from build123d import *

# Parameters (mm, degrees)
LEFT_EXT_DEPTH = 63.5
HOLE_R         = 4.699
HOLE_CUT_DEPTH = 286.961588331


with BuildPart() as part:
    # Left → left_ext (new body)
    with BuildSketch(Plane.XY):
        Polygon((-165.1, 19.05), (-10.998522627, 285.961588331), (10.998522629, 285.961588331), (-143.102954744, 19.05), align=None)
    extrude(amount=LEFT_EXT_DEPTH)

    # hole → hole_cut (cut, through all)
    with BuildSketch(Plane(origin=(0, 0, 0), x_dir=(1, 0, 0), z_dir=(0, 1, 0))):
        with Locations((0, -31.75)):
            Circle(HOLE_R)
    extrude(amount=HOLE_CUT_DEPTH, mode=Mode.SUBTRACT)


solid = part.part
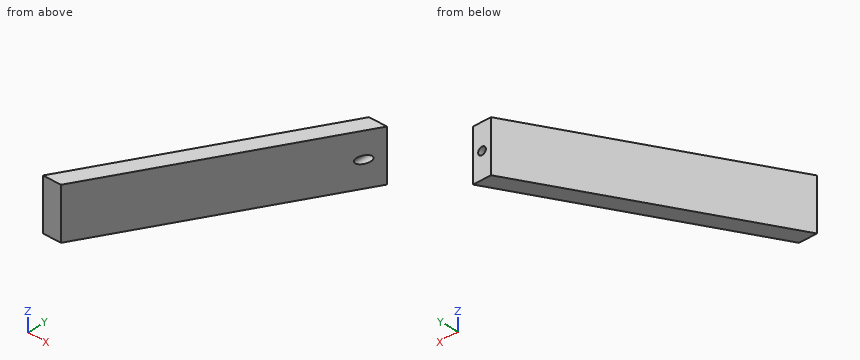
For this review, take the finished solid that the model builds, in its own axes (mm). Coordinates: 2 decimals unless noted, no trailing zeros. Loops run counter-clockwise (first coordinate to the right, second up) from the corner with the lowest first, then second, coordinate; pieces in that order, holes last. Notation, with made-up numbers: (-5, -24.5) - (4, -24.5) arc R38 ccw to (4, 14.5) - close; hole circle Ø5 at (-9, 78.5). An arc over 180 degrees is marked (long way). Return JSON: item names as keys, results as strings.
Item 1: Insertion check: pin 1 (8.5 mm diameter, centred on x = 0, z = 31.75, fed in from -Y); pin 2 (2 mm diameter, centred on y = 233, z = 34, fed in from -X); pin 3 (8 mm diameter, centred on x = -129, z = 27.5, fed in from +Y); pin 4 (4 mm diameter, centred on y = 74.5, z = 13.5, fed in from -X). Each pin has a flat end and moves straight along its axis. Give the tip position at first contact, or say it passes through.
Determined:
{"pin 1": "passes through", "pin 2": "stops at x = -42.15", "pin 3": "stops at y = 88.51", "pin 4": "stops at x = -134.24"}
Item 2: For line 1 (Z direction, x = 0, y = 269); line 2 (Y direction, x = -133.5, z = 11); line 3 (X direction, y = 49.5, z = 8), list the stretches that pass through material, from the lowest coordinate up.
Determined:
{"line 1": "z = 0 to 27.05, 36.45 to 63.5", "line 2": "y = 35.68 to 73.78", "line 3": "x = -147.52 to -125.52"}
Item 3: Take a section at D-D (y = 107.5). Give the boundary of the cut face in (x, z).
Determined:
{"outline": "(-114.03, 0) - (-92.04, 0) - (-92.04, 63.5) - (-114.03, 63.5) - close"}
Item 4: Take a section at A-A (z = 31.75). Give the boundary of the cut face in (x, y).
Determined:
{"outline": "(-165.1, 19.05) - (-143.1, 19.05) - (-4.7, 258.77) - (-4.7, 285.96) - (-11, 285.96) - close; (4.7, 275.05) - (11, 285.96) - (4.7, 285.96) - close"}
Item 5: Take a section at B-B (x = 0). Give the boundary of the cut face in (y, z), then the cut area to 3 significant figures.
Determined:
{"outline": "(266.91, 0) - (285.96, 0) - (285.96, 27.05) - (266.91, 27.05) - close; (266.91, 36.45) - (285.96, 36.45) - (285.96, 63.5) - (266.91, 63.5) - close", "area": "1,030 mm2"}
Item 6: Take a section at C-C (z = 7.5). Give the boundary of the cut face in (x, y), then the cut area to 3 significant figures.
Determined:
{"outline": "(-165.1, 19.05) - (-143.1, 19.05) - (11, 285.96) - (-11, 285.96) - close", "area": "5,870 mm2"}
